Verification items for the finished model (mm, model axes). Face numbers are marked on the shaded views. Round coordinates to 2 decimals unless told otherwise and drop trailing zeros. Write each loop counter-clockwise with the first axis right and the second up, starting at its lowest first coordinate (ties: lowest second). Pieces come first, ordered by that corner, then holes. Notation, with made-up numbers: M -40,26 L -24,26 A36 ccw -24,60 Z; hole C -19.75,79 d9. An arc over 180 degrees is marked long. One line per item, written item: value. Start each with the question number.
Item 1: Thickness scan on probe 1 along Y at (x, z) = (-8, 1.5); probe 2 along X at (y, z) = (-4.75, 1.05); probe 3 along Y at (x, z) = (-10, 1.95). Record the ranges inside material, lowest first. Write a range as from..to.
Item 2: Section check B-B, the plane x = 12.5. Record the cut outline in (y, z).
Item 3: Gauge pin test, flat end, axial feed: pin 1 (1.5 mm diameter, centred on x = -8, y = 0.5, fed in from -Z). Record the tip position at first contact, or that the pin passes through.
Item 4: Section check D-D, the plane x = 1. Record the cut outline in (y, z), then the cut area to 3 significant figures.
Item 5: Section check C-C, the plane x = 8. Record the cut outline in (y, z), then the cut area to 3 significant figures.
Item 6: Draft check along Y on the marked faces 1, 2, 3 and 4. Enter one of: +Y half, -Y half, draft (parallel to the pull), parting line (faces both ways), or undercut.
from build123d import *

# Parameters (mm, degrees)
F0_W     = 32
F0_H     = 16
F1_DEPTH = 3
F2_W     = 29
F2_H     = 13
F2_R     = 3.25
F2_R_2   = 2.5
F3_DEPTH = 2


with BuildPart() as f1:
    # F0 (on Top) → F1 (new body)
    with BuildSketch(Plane.XY):
        Rectangle(F0_W, F0_H)
    extrude(amount=F1_DEPTH)

    # F2 (on face) → F3 (cut)
    with BuildSketch(Plane(origin=(0, 0, 0), x_dir=(1, 0, 0), z_dir=(0, 0, -1))):
        Rectangle(F2_W, F2_H)
        with Locations((-8, 0)):
            Circle(F2_R, mode=Mode.SUBTRACT)
        Circle(F2_R, mode=Mode.SUBTRACT)
        with Locations((8, 0)):
            Circle(F2_R, mode=Mode.SUBTRACT)
        with Locations((-8, 0)):
            Circle(F2_R_2)
        Circle(F2_R_2)
        with Locations((8, 0)):
            Circle(F2_R_2)
    extrude(amount=-F3_DEPTH, mode=Mode.SUBTRACT)


solid = f1.part
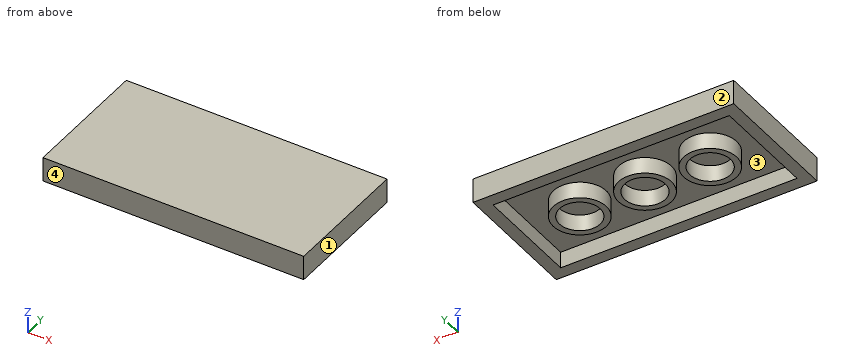
Response values:
1. probe 1: y = -8..-6.5, -3.25..-2.5, 2.5..3.25, 6.5..8
1. probe 2: x = -16..-14.5, 14.5..16
1. probe 3: y = -8..-6.5, -2.56..-1.5, 1.5..2.56, 6.5..8
2. outline: M -8,0 L -6.5,0 L -6.5,2 L 6.5,2 L 6.5,0 L 8,0 L 8,3 L -8,3 Z
3. pin 1: stops at z = 2
4. outline: M -8,0 L -6.5,0 L -6.5,2 L -3.09,2 L -3.09,0 L -2.29,0 L -2.29,2 L 2.29,2 L 2.29,0 L 3.09,0 L 3.09,2 L 6.5,2 L 6.5,0 L 8,0 L 8,3 L -8,3 Z
4. area: 25.2 mm2
5. outline: M -8,0 L -6.5,0 L -6.5,2 L -3.25,2 L -3.25,0 L -2.5,0 L -2.5,2 L 2.5,2 L 2.5,0 L 3.25,0 L 3.25,2 L 6.5,2 L 6.5,0 L 8,0 L 8,3 L -8,3 Z
5. area: 25.0 mm2
6. face 1: draft
6. face 2: +Y half
6. face 3: undercut
6. face 4: -Y half
